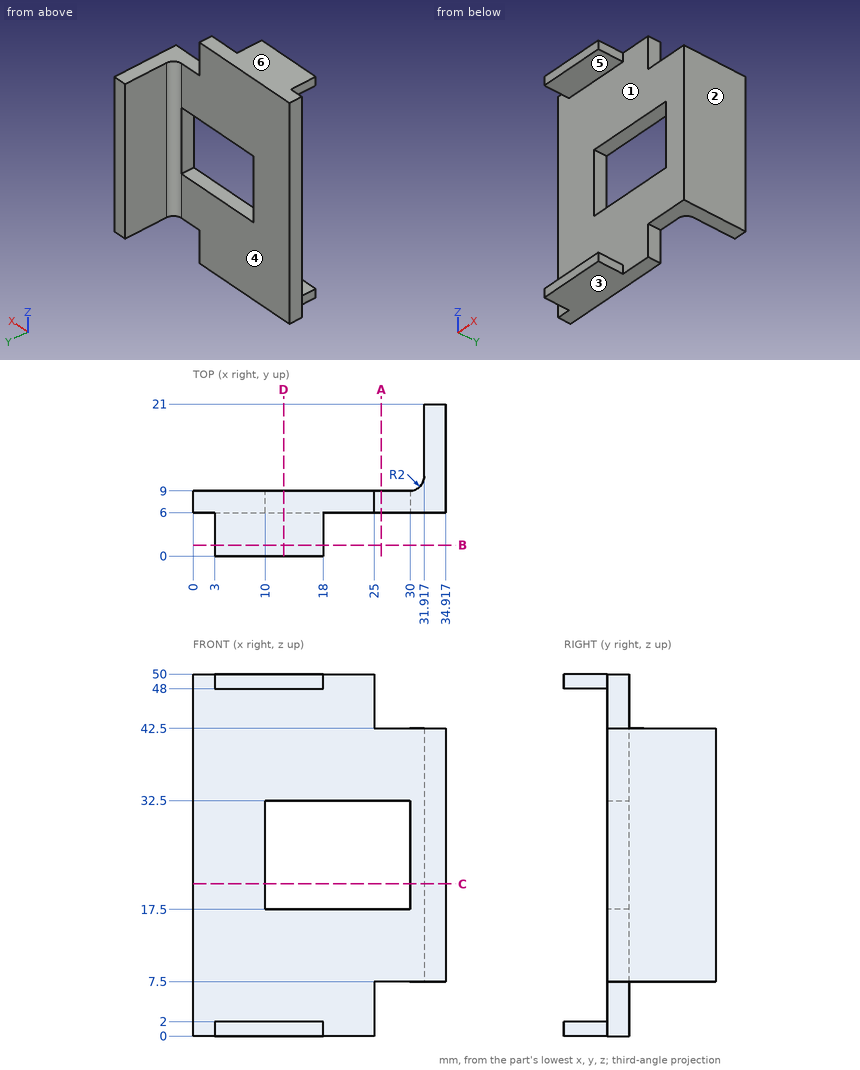
Part print with two shaded views. Sizes in mm from the minimum x, y, z corner. A direction names the side the tool comes from. Coordinates: 2 decimals unless noted, no trailing zeros. Write each loop counter-clockwise with the first axis right and the second up, starting at its lowest first coordinate (ties: lowest second). Pieces come first, ordered by that corner, then holes. Notation, with made-up numbers: (28, -11) - (80, -11) arc R30 cw to (80, 19) - close; hole circle Ø4 at (37.25, 71.25). An arc over 180 degrees is marked (long way). Use a Markdown table: item, result. Add a question column.
Item 1: Drill centre lines: line 1 along Z through (x, y) = (28, 7.25); line 2 along X through (y, z) = (8.25, 25); line 3 along Z through (x, y) = (17, 8.5). Where is each one in solid material? Low to high.
Item 2: Band-saw the part on C-C, the plane z = 21. Write the cut outline in (x, y), and give its area (3 significant figures).
Item 3: 3-axis set-ups, long thin cutter, end or side, ignore diameter. For the marked faces 4, 5 and 6: which of +Z, -Z, +X, -X, +Y, -Y reach the whole face in a straight line?
Item 4: Two-plate mould, pull along Z, no slides. Class the marked faces 1, 2 and 3: pulls with the +Z half, pulls with the -Z half, needs draft (parallel to the pull), parting line crosses it, or undercut.
Item 5: Drop flat-ended pins along their axis: pin 1 (8 mm diameter, centred on x = 25.5, z = 38.5, fed in from -Y); pin 2 (6 mm diameter, centred on y = 13, z = 10.5, fed in from -X); pin 3 (5 mm diameter, centred on x = 31, y = 10.5, fed in from -Z); pin 4 (3 mm diameter, centred on x = 14, y = 4, fed in from -Z). Give the stop position or say it passes through.
Item 6: Band-saw the part on B-B, the plane y = 1.5. Write the cut outline in (x, z).
Item 7: Band-saw the part on D-D, the plane x = 12.5. Write the cut outline in (y, z), and give its area (3 significant figures).
Item 8: Band-saw the part on A-A, the plane x = 26. Write the cut outline in (y, z).
A:
| question | item | result |
|---|---|---|
| 1 | line 1 | z = 7.5 to 17.5, 32.5 to 42.5 |
| 1 | line 2 | x = 0 to 10, 30 to 34.92 |
| 1 | line 3 | z = 0 to 17.5, 32.5 to 50 |
| 2 | outline | (0, 6) - (10, 6) - (10, 9) - (0, 9) - close; (30, 6) - (34.92, 6) - (34.92, 21) - (31.92, 21) - (31.92, 11) arc R2 cw to (30, 9) - close |
| 2 | area | 81.6 mm² |
| 3 | face 4 | +Z, -Z, -X, +Y |
| 3 | face 5 | +X, -X, -Y |
| 3 | face 6 | +Z, +X, -X, +Y, -Y |
| 4 | face 1 | undercut |
| 4 | face 2 | needs draft |
| 4 | face 3 | pulls with the -Z half |
| 5 | pin 1 | stops at y = 6 |
| 5 | pin 2 | stops at x = 31.65 |
| 5 | pin 3 | stops at z = 7.5 |
| 5 | pin 4 | stops at z = 0 |
| 6 | outline | (3, 0) - (18, 0) - (18, 2) - (3, 2) - close; (3, 48) - (18, 48) - (18, 50) - (3, 50) - close |
| 7 | outline | (0, 0) - (9, 0) - (9, 17.5) - (6, 17.5) - (6, 2) - (0, 2) - close; (0, 48) - (6, 48) - (6, 32.5) - (9, 32.5) - (9, 50) - (0, 50) - close |
| 7 | area | 129 mm² |
| 8 | outline | (6, 7.5) - (9, 7.5) - (9, 17.5) - (6, 17.5) - close; (6, 32.5) - (9, 32.5) - (9, 42.5) - (6, 42.5) - close |
